Answer from the drawing. Dimensions are ordinates in mm from the lowest x, y and z of the part. A direction names the side the tool comes from. Give positions to 0.01 mm unless a question says otherwise; leave off trailing zeros. Order: outer loops, then holes, each group sorted by start corner. A loop starts at its lowest first (then second) coordinate and runs counter-clockwise, first axis right, second up. Notation, with made-up numbers: (32.25, 7) -> (61.25, 7) arc R31 ccw to (61.25, 46) -> close; hole circle Ø4 at (74, 40.5). An arc over 180 degrees is marked (long way). Answer as CSV lines item,"result". Start each with the question number.
1) Flat-ended cylindrical pins translate along their axes: pin 1 Ø6 at (y, z) = (11, 8) entering from -X; pin 2 Ø0.8 at (x, z) = (24.5, 9.5) entering from -Y; pin 3 Ø2.5 at (x, z) = (26, 1) entering from +Y; pin 4 Ø1 at (x, z) = (10.5, 5) entering from -Y. Find the tip coordinate at first contact, or state that the pin passes through.
2) The mould has two halves that part along X. Classify the marked faces 1, 2 and 3: +X half, -X half, draft (parallel to the pull), parting line (faces both ways), or undercut.
3) For the marked faces 4, 5, 6 and 7, determine the directions among +Z, -Z, +X, -X, +Y, -Y from which every point of the face is accessible in a straight line to the end or side of a thin tool.
4) Straight lines are drawn through the part: L1, parallel to Y at x = 10, z = 2.4; L2, parallel to Y at x = 26.5, z = 13; L3, parallel to Y at x = 14.75, z = 8. For each, find the intervals that lie inside material, in ascending order. Write a range as from..to.
5) Find section C-C (x = 2.5). Determine the outline of the cut face in (y, z), and give its area (3 significant figures).
6) Find section A-A (z = 5). Determine the outline of the cut face in (x, y), and give its area (3 significant figures).
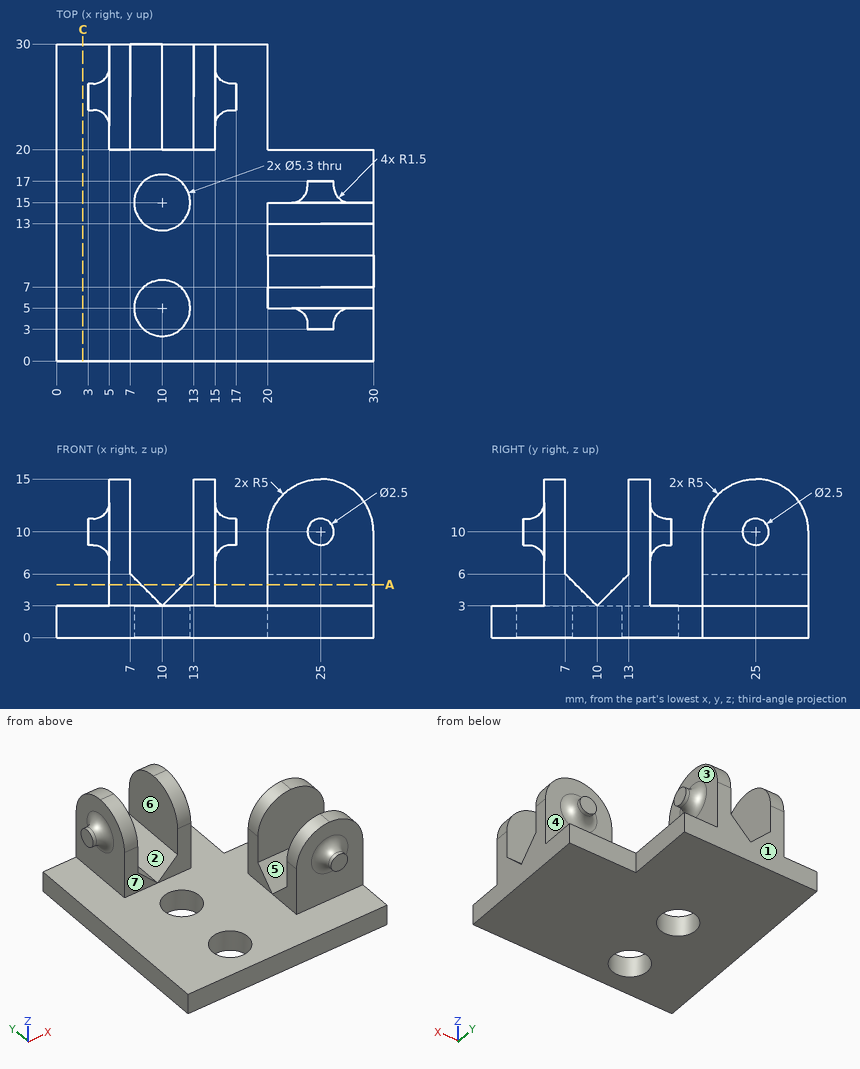
Findings below:
1,pin 1,"x = 20"
1,pin 2,"y = 3"
1,pin 3,"y = 20"
1,pin 4,"through"
2,face 1,"draft"
2,face 2,"undercut"
2,face 3,"+X half"
3,face 4,"+Y"
3,face 5,"+Z, +X, -X"
3,face 6,"+Z, +Y, -Y"
3,face 7,"+Z, +X, -X, -Y"
4,L1,"0..2.35, 7.65..12.35, 17.65..30"
4,L2,"5..7, 13..15"
4,L3,"20..30"
5,outline,"(0, 0) -> (30, 0) -> (30, 3) -> (0, 3) -> close"
5,area,"90.0 mm²"
6,outline,"(5, 20) -> (8, 20) -> (8, 30) -> (5, 30) -> close; (12, 20) -> (15, 20) -> (15, 30) -> (12, 30) -> close; (20, 5) -> (30, 5) -> (30, 8) -> (20, 8) -> close; (20, 12) -> (30, 12) -> (30, 15) -> (20, 15) -> close"
6,area,"120 mm²"
